Design review of the part built by this model. Coordinates are the model's own, in mm. A direction names the side the tool comes from. Give positions to 0.01 mm unless a question says otherwise; leave off trailing zeros. Loops run counter-clockwise (first coordinate to the right, second up) from the corner with the lowest first, then second, coordinate; pieces in that order, holes last. Notation, with made-up numbers: M 86,-33.75 L 131,-33.75 A30 ccw 131,-3.75 Z; hole C -22,5.5 d1. An arc over 180 degrees is marked long. Use a Markdown table: item, result. Add a question column.
(1) Add section B-B, the plane z = 60. Give the boundary of the cut face in (x, y).
(2) Add section C-C, the plane x = 0. Give the boundary of the cut face in (y, z).
(3) For faces 4 (the face through (0, -1, 80)), 5 (the face through (0, -1, 84)), list the 3-axis set-ups (+Z, -Z, +X, -X, +Y, -Y) from which the entire face can be reached by the end or side of a thin tool; tool diameter is ignored.
(4) Add section A-A, the plane y = -0.65. Give the boundary of the cut face in (x, z), then the cut area to 3 significant figures.
(5) For probe 1 along Z at (x, y) = (0, -0.7); probe 2 along X at (y, z) = (-0.1, 69); probe 3 along Z at (x, y) = (-0.5, -1.7), list the stretches that pass through material, from the lowest coordinate up.
(6) Draft analysis for pull direction X (two halves, no side actions). For faces 1 (the face through (1, -1, 67)), 2 (the face through (0, 0, 40)), 3 (the face through (-5, -1, 40)), state which applies: pulls with the +X half, pulls with the -X half, needs draft (parallel to the pull), parting line crosses it, or undercut.
(7) Add section D-D, the plane z = 51. Give the boundary of the cut face in (x, y).
```python
from build123d import *

# Parameters (mm, degrees)
F0_R     = 2
F1_DEPTH = 3


with BuildPart() as f1:
    # F0 (on Front) → F1 (new body)
    with BuildSketch(Plane.XZ):
        with BuildLine():
            Line((-5, 79), (-5, 0))
            ThreePointArc((-5, 0), (0, -5), (5, 0))
            Line((5, 0), (5, 79))
            ThreePointArc((5, 79), (0, 84), (-5, 79))
        make_face()
        with Locations((0, 51)):
            Circle(F0_R, mode=Mode.SUBTRACT)
        with BuildLine():
            ThreePointArc((-1, 79), (0, 80), (1, 79))
            Line((1, 79), (1, 55))
            ThreePointArc((1, 55), (0, 54), (-1, 55))
            Line((-1, 55), (-1, 79))
        make_face(mode=Mode.SUBTRACT)
    extrude(amount=F1_DEPTH)


solid = f1.part
```
Established:
| question | item | result |
|---|---|---|
| 1 | outline | M -5,-3 L -1,-3 L -1,0 L -5,0 Z; M 1,-3 L 5,-3 L 5,0 L 1,0 Z |
| 2 | outline | M -3,-5 L 0,-5 L 0,49 L -3,49 Z; M -3,53 L 0,53 L 0,54 L -3,54 Z; M -3,80 L 0,80 L 0,84 L -3,84 Z |
| 3 | face 4 | +Y, -Y |
| 3 | face 5 | +Z, +Y, -Y |
| 4 | outline | M -5,0 A5 ccw 5,0 L 5,79 A5 ccw -5,79 Z; hole C 0,51 d4; hole M -1,55 A1 ccw 1,55 L 1,79 A1 ccw -1,79 Z |
| 4 | area | 805 mm^2 |
| 5 | probe 1 | -5 to 49, 53 to 54, 80 to 84 |
| 5 | probe 2 | -5 to -1, 1 to 5 |
| 5 | probe 3 | -4.97 to 49.06, 52.94 to 54.13, 79.87 to 83.97 |
| 6 | face 1 | undercut |
| 6 | face 2 | needs draft |
| 6 | face 3 | pulls with the -X half |
| 7 | outline | M -5,-3 L -2,-3 L -2,0 L -5,0 Z; M 2,-3 L 5,-3 L 5,0 L 2,0 Z |
